Can you work these out from the model? Positions are in its coordinate system, mm. Give positions to 0.01 mm unless a question says otherwise; leave off trailing zeros. Order: outer loops, then holes, each group sorted by start corner. A loop starts at its lowest first (then second) coordinate and runs counter-clockwise, first axis right, second up. Notation, with made-up numbers: (62, 52) - (81, 52) arc R19 ccw to (81, 82) - close; hole circle Ø9 at (-29.75, 36). An arc over 180 degrees is marked (long way). Answer as CSV lines item,"result".
Autodesk Inventor part; units mm, degrees
ref_plane "YZ Plane" through (0, 0, 0) normal (1, 0, 0) x (0, 1, 0)
ref_plane "XZ Plane" through (0, 0, 0) normal (0, 1, 0) x (-1, 0, 0)
ref_plane "XY Plane" through (0, 0, 0) normal (0, 0, 1) x (1, 0, 0)
sketch "Boceto1" plane through (0, 0, 0) normal (0, 0, 1) x (1, 0, 0)
  arc A0 (0, 5) -> (0, -5) centre (0, 0) ccw
  arc A1 (170, -5) -> (170, 5) centre (170, 0) ccw
  line L0 (0, 5) -> (170, 5)
  line L1 (0, -5) -> (170, -5)
  circle A2 centre (0, 0) radius 2.5
  circle A3 centre (170, 0) radius 2.5
  circle A4 centre (85, 0) radius 2.5
  dimension "d1" = 10
  dimension "d2" = 10
  dimension "d3" = 5
  dimension "d4" = 5
  dimension "d8" = 5
  dimension "d11" = 85
  dimension "d12" = 85
extrude "Extrusión1" add sketch "Boceto1" along normal blind 5
properties part number "Eslabon2"
1) If we mould it in two halves opening along Y, with no side actions, what happens to faces 1 (the flat face through (84, 3, 0)), 2 (the flat face through (84, -5, 2)), 3 (the cylindrical face through (-0.54, 2.44, 2.46))? For each: +Y half, -Y half, draft (parallel to the pull), parting line (faces both ways), or undercut.
Answer block:
face 1,"draft"
face 2,"-Y half"
face 3,"undercut"
2) I'm going to push flat-ended pins straight in: P1, Ø2, axis at y = 1.5, z = 1, coming from the -X side; P2, Ø3, axis at x = 0, y = 0, coming from the -Z side; P3, Ø3, axis at y = 3.5, z = 2, coming from the -X side. Where does each tip first touch, or does it pass through?
Answer block:
P1,"x = -4.97"
P2,"through"
P3,"x = -4.58"
3) I want a section at C-C on x = 85. Write out the boundary of the cut face in (y, z).
Answer block:
outline,"(-5, 0) - (-2.5, 0) - (-2.5, 5) - (-5, 5) - close; (2.5, 0) - (5, 0) - (5, 5) - (2.5, 5) - close"
4) I want a section at B-B on z = 2.4. Write out the boundary of the cut face in (x, y).
Answer block:
outline,"(0, -5) - (170, -5) arc R5 ccw to (170, 5) - (0, 5) arc R5 ccw to start; hole circle Ø5 at (0, 0); hole circle Ø5 at (85, 0); hole circle Ø5 at (170, 0)"
5) I want a section at A-A on y = 0. Write out the boundary of the cut face in (x, z), plus the area to 3 significant figures.
Answer block:
outline,"(-5, 0) - (-2.5, 0) - (-2.5, 5) - (-5, 5) - close; (2.5, 0) - (82.5, 0) - (82.5, 5) - (2.5, 5) - close; (87.5, 0) - (167.5, 0) - (167.5, 5) - (87.5, 5) - close; (172.5, 0) - (175, 0) - (175, 5) - (172.5, 5) - close"
area,"825 mm2"
6) I need wall thicknesses on line 1 along Y through (x, z) = (85, 1.5); line 2 along X through (y, z) = (-2, 1.7); line 3 along X through (y, z) = (0.75, 2.7). Which ranges of each line are inside material? Lowest first, please. Write a range as [from, to].
Answer block:
line 1,"[-5, -2.5], [2.5, 5]"
line 2,"[-4.58, -1.5], [1.5, 83.5], [86.5, 168.5], [171.5, 174.58]"
line 3,"[-4.94, -2.38], [2.38, 82.62], [87.38, 167.62], [172.38, 174.94]"
